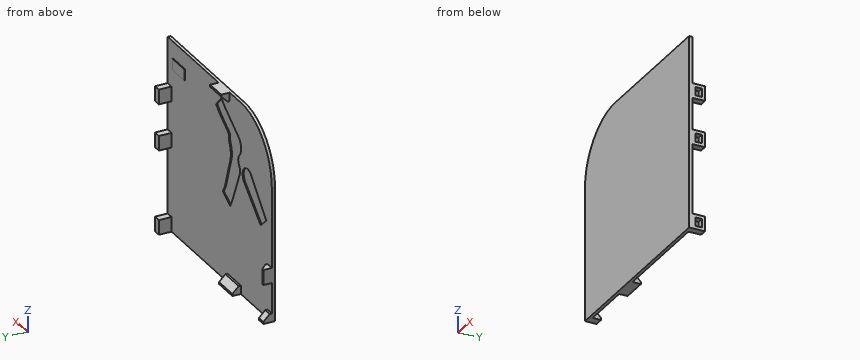
from build123d import *

# Parameters (mm, degrees)
EXTRUDE_1_DEPTH     = 1.5
SKETCH_3_W          = 7
SKETCH_3_H          = 6
SKETCH_3_W_2        = 4
SKETCH_3_H_2        = 3
EXTRUDE_3_DEPTH     = 3
SKETCH_4_W          = 7
SKETCH_4_H          = 6
EXTRUDE_4_DEPTH     = 0.5
SKETCH_5_W          = 4
SKETCH_5_H          = 4
SKETCH_5_W_2        = 12
SKETCH_5_H_2        = 7.145089785
SKETCH_5_W_3        = 10
EXTRUDE_5_DEPTH     = 4
CHAMFER_1_SIZE      = 3
CUT_EXTRUDE_2_DEPTH = 0.5
SKETCH_8_W          = 10.8
SKETCH_8_H          = 5.3
EXTRUDE_6_DEPTH     = 1.85


with BuildPart() as part:
    # Эскиз1 → Бобышка-Вытянуть1 (new body)
    with BuildSketch(Plane(origin=(0, 0, 0), x_dir=(1, 0, 0), z_dir=(0, 1, 0))):
        with BuildLine():
            Line((-27.5, 63.5), (-27.5, 0))
            ThreePointArc((-27.5, 0), (-19.445436483, -19.445436483), (0, -27.5))
            Line((0, -27.5), (66.5, -27.5))
            Line((66.5, -27.5), (66.5, 63.5))
            Line((66.5, 63.5), (-27.5, 63.5))
        make_face()
    extrude(amount=EXTRUDE_1_DEPTH)

    # Эскиз3 → Бобышка-Вытянуть3 (add)
    # profile 1 of 3: a face of its own
    with BuildSketch(Plane(origin=(66.5, 0, 0), x_dir=(0, 0, -1), z_dir=(1, 0, 0))):
        with Locations((-2, 4.5)):
            Rectangle(SKETCH_3_W, SKETCH_3_H)
        with Locations((-2, 4.5)):
            Rectangle(SKETCH_3_W_2, SKETCH_3_H_2, mode=Mode.SUBTRACT)
    # profile 2 of 3: a face of its own
    with BuildSketch(Plane(origin=(66.5, 0, 0), x_dir=(0, 0, -1), z_dir=(1, 0, 0))):
        with Locations((60, 4.5)):
            Rectangle(SKETCH_3_W, SKETCH_3_H)
        with Locations((60, 4.5)):
            Rectangle(SKETCH_3_W_2, SKETCH_3_H_2, mode=Mode.SUBTRACT)
    # profile 3 of 3: a face of its own
    with BuildSketch(Plane(origin=(66.5, 0, 0), x_dir=(0, 0, -1), z_dir=(1, 0, 0))):
        with Locations((20, 4.5)):
            Rectangle(SKETCH_3_W, SKETCH_3_H)
        with Locations((20, 4.5)):
            Rectangle(SKETCH_3_W_2, SKETCH_3_H_2, mode=Mode.SUBTRACT)
    extrude(amount=-EXTRUDE_3_DEPTH)

    # Эскиз4 → Бобышка-Вытянуть4 (add)
    with BuildSketch(Plane.ZY.offset(-63.5)):
        with Locations((-60, 4.5)):
            Rectangle(SKETCH_4_W, SKETCH_4_H)
        with Locations((-20, 4.5)):
            Rectangle(SKETCH_4_W, SKETCH_4_H)
        with Locations((2, 4.5)):
            Rectangle(SKETCH_4_W, SKETCH_4_H)
    extrude(amount=EXTRUDE_4_DEPTH)

    # Эскиз5 → Бобышка-Вытянуть5 (add)
    with BuildSketch(Plane(origin=(0, 1.5, 0), x_dir=(1, 0, 0), z_dir=(0, 1, 0))):
        with Locations((-25.5, 61.5)):
            Rectangle(SKETCH_5_W, SKETCH_5_H)
        with Locations((6.5, 61.5)):
            Rectangle(SKETCH_5_W_2, SKETCH_5_H)
        with Locations((-25.5, 41.427455108)):
            Rectangle(SKETCH_5_W, SKETCH_5_H_2)
        with Locations((15.5, -25.5)):
            Rectangle(SKETCH_5_W_3, SKETCH_5_H)
    extrude(amount=EXTRUDE_5_DEPTH)

    # Фаска1
    chamfer_1_edges = [part.edges().sort_by_distance(p)[0] for p in [
        (6.5, 5.5, -59.5),
        (-25.5, 5.5, -59.5),
        (-23.5, 5.5, -41.427455107),
        (15.5, 5.5, 23.5),
    ]]
    chamfer(chamfer_1_edges, length=CHAMFER_1_SIZE)

    # Эскиз7 → Вырез-Вытянуть2 (cut)
    with BuildSketch(Plane(origin=(0, 1.5, 0), x_dir=(1, 0, 0), z_dir=(0, 1, 0))):
        with BuildLine():
            Line((-19.62312526, 14.49129531), (-22.541249894, 17.745613481))
            Line((-22.541249894, 17.745613481), (-17.469363806, 22.293538718))
            Line((-17.469363806, 22.293538718), (-14.49129531, 19.62312526))
            Line((-14.49129531, 19.62312526), (-2.655568985, 9.010111183))
            ThreePointArc((-2.655568985, 9.010111183), (-2.47780361, 2.47780361), (-9.010111183, 2.655568985))
            Line((-9.010111183, 2.655568985), (-19.62312526, 14.49129531))
        make_face()
        with BuildLine():
            Line((9.950995869, 4.304852328), (14.772590148, 18.914824353))
            Line((14.772590148, 18.914824353), (16.702744877, 22.418322994))
            Line((16.702744877, 22.418322994), (10.02542163, 26.097007748))
            Line((10.02542163, 26.097007748), (8.095266902, 22.593509107))
            Line((8.095266902, 22.593509107), (1.302167241, 6.782804644))
            ThreePointArc((1.302167241, 6.782804644), (1.249533327, 4.765531423), (2.083776147, 2.928087411))
            ThreePointArc((2.083776147, 2.928087411), (2.810034737, 0.519874571), (1.770696829, -1.770696829))
            ThreePointArc((1.770696829, -1.770696829), (0.184130493, -6.176714777), (2.567220604, -10.207976169))
            Line((2.567220604, -10.207976169), (15.04943055, -18.695310645))
            Line((15.04943055, -18.695310645), (17.989670533, -21.407318912))
            Line((17.989670533, -21.407318912), (22.788067369, -16.205108284))
            Line((22.788067369, -16.205108284), (19.847827385, -13.493100017))
            Line((19.847827385, -13.493100017), (12.232446688, -8.314987854))
            ThreePointArc((12.232446688, -8.314987854), (11.3870962, -7.335158785), (11.144915737, -6.063926675))
            ThreePointArc((11.144915737, -6.063926675), (11.047783222, -4.555489901), (10.543689128, -3.130461702))
            ThreePointArc((10.543689128, -3.130461702), (9.497003398, 0.527383324), (9.950995869, 4.304852328))
        make_face()
    extrude(amount=-CUT_EXTRUDE_2_DEPTH, mode=Mode.SUBTRACT)

    # Эскиз8 → Бобышка-Вытянуть6 (add)
    with BuildSketch(Plane(origin=(0, 0, 0), x_dir=(1, 0, 0), z_dir=(0, 1, 0))):
        with Locations((56.1, -16.85)):
            Rectangle(SKETCH_8_W, SKETCH_8_H)
    extrude(amount=EXTRUDE_6_DEPTH)


solid = part.part
Geometry: final body of the model. Coordinates: model frame, mm. Give positions to 0.01 mm unless a question says otherwise; leave off trailing zeros. Loops run counter-clockwise (first coordinate to the right, second up) from the corner with the lowest first, then second, coordinate; pieces in that order, holes last. Notation, with made-up numbers: M 18,26.25 L 74,26.25 A10 ccw 74,43.25 Z; hole C 82.25,-18 d7. An arc over 180 degrees is marked long. Put each result on its own line as item: value. Start each with the question number.
1) Cut plane A-A (z = -41.5). Output: boundary loops of the cut face in (x, y), then the cut area to 4 significant figures.
2) Cut plane B-B (x = -6.5). Output: boundary loops of the cut face in (y, z).
3) Contact query for flat-ended pins moving along their axis: pin 1 (0.9 mm diameter, centred on y = 5, z = 1.5, fed in from +X); pin 2 (1.8 mm diameter, centred on x = 64.5, y = 5.5, fed in from +Z); pin 3 (2 mm diameter, centred on y = 3, z = 26.5, fed in from +X); pin 4 (1.1 mm diameter, centred on x = 14.5, y = 2, fed in from -Z). Output: stop coordinate, or through.
4) Cut plane C-C (x = 46). Output: boundary loops of the cut face in (y, z), then the cut area to 4 significant figures.
5) Ray query, line 1 along Y through (x, z) = (51, 21); line 2 along Z through (x, y) = (4.5, 3.5); line 3 along Z through (x, y) = (13, 5). Return the intervals inside material, ascending.
6) Cut plane D-D (z = -29.5). Output: boundary loops of the cut face in (x, y).
Verdict:
1. outline: M -27.5,0 L 66.5,0 L 66.5,1.5 L -23.5,1.5 L -23.5,2.5 L -26.5,5.5 L -27.5,5.5 Z
1. area: 152.5 mm2
2. outline: M 0,-63.5 L 1.5,-63.5 L 1.5,-12.46 L 1,-12.46 L 1,-1.24 L 1.5,-1.24 L 1.5,26.72 L 0,26.72 Z
3. pin 1: x = 63.5
3. pin 2: z = 5.5
3. pin 3: x = 20.5
3. pin 4: z = -63.5
4. outline: M 0,-63.5 L 1.5,-63.5 L 1.5,27.5 L 0,27.5 Z
4. area: 136.5 mm2
5. line 1: 0 to 1.5
5. line 2: -63.5 to -60.5
5. line 3: 26 to 27.5
6. outline: M -27.5,0 L 66.5,0 L 66.5,1.5 L -27.5,1.5 Z
